from build123d import *

# Parameters (mm, degrees)
F0_W      = 101.61
F0_H      = 146
F1_DEPTH  = 1
F3_W      = 2
F3_H      = 146
F3_H_2    = 43.5
F4_DEPTH  = 9
F5_W      = 97.61
F5_H      = 5
F6_DEPTH  = 3
F9_W      = 5.5
F9_H      = 6
F10_DEPTH = 9
F11_D     = 2.7051
F12_D     = 3.7973


with BuildPart() as f1:
    # F0 (on Top) → F1 (new body)
    with BuildSketch(Plane.XY):
        with Locations((-50.805, -73)):
            Rectangle(F0_W, F0_H)
    extrude(amount=-F1_DEPTH)

    # F3 (on Top) → F4 (join)
    with BuildSketch(Plane.XY):
        with Locations((-100.61, -73)):
            Rectangle(F3_W, F3_H)
        with Locations((-1, -124.25)):
            Rectangle(F3_W, F3_H_2)
    extrude(amount=F4_DEPTH)

    # F5 (on face) → F6 (join)
    with BuildSketch(Plane.XY):
        with Locations((-50.805, -105)):
            Rectangle(F5_W, F5_H)
    extrude(amount=F6_DEPTH)

    # F9 (on face) → F10 (join, through all)
    with BuildSketch(Plane.XY):
        with Locations((-98.86, -130.3)):
            Rectangle(F9_W, F9_H)
        with Locations((-98.86, -70.11)):
            Rectangle(F9_W, F9_H)
        with Locations((-98.86, -28.5)):
            Rectangle(F9_W, F9_H)
        with Locations((-2.75, -130.3)):
            Rectangle(F9_W, F9_H)
    extrude(amount=F10_DEPTH)

    # F11 (through all)
    with Locations(Plane(origin=(-101.61, 0, 0), x_dir=(0, -1, 0), z_dir=(-1, 0, 0))):
        with Locations((28.5, 5.35), (70.11, 5.35), (130.3, 5.35)):
            Hole(F11_D / 2)

    # F12 (through all)
    with Locations(Plane.XY):
        with Locations((-65.785, -90.6), (-4.065, -90.6), (-4.065, -14), (-65.785, -14)):
            Hole(F12_D / 2)


solid = f1.part
The model under review builds one solid part; all positions refer to its coordinate system, in mm. A direction names the side the tool comes from. Round coordinates to 2 decimals unless told otherwise and drop trailing zeros. Order: outer loops, then holes, each group sorted by start corner. A loop starts at its lowest first (then second) coordinate and runs counter-clockwise, first axis right, second up. Notation, with made-up numbers: (-20.75, 56.5) -> (31.25, 56.5) arc R26 cw to (31.25, 70.5) -> close; hole circle Ø1 at (77, 45.5). An arc over 180 degrees is marked (long way). Use CSV: the item, a comma, the result in double quotes. Start each with the question number.
(1) Consider section B-B on x = -65.5. Write out the cut boundary in (y, z).
(2) Consider section C-C on y = -112. Write out the cut boundary in (x, z), and give its area (3 significant figures).
(3) Tool access review of faces 5 (the face through (-98, -73.11, 4)), 6 (the face through (-98, -25.5, 4)), 7 (the face through (-2, -115, 4)): name each direction out of +Z, -Z, +X, -X, +Y, -Y from which nothing blocks a thin tool from reaching the whole face with its end or side.
(4) Insertion check: pin 1 (1.5 mm diameter, centred on y = -76, z = 8, fed in from +X); pin 2 (3.5 mm diameter, centred on y = -130.3, z = 5.35, fed in from +X); pin 3 (1 mm diameter, centred on x = -97.5, z = 3.5, fed in from +Y); pin 4 (2.5 mm diameter, centred on y = -70.11, z = 5.35, fed in from +X). Each pin has a flat end and moves straight along its axis. Give the tip position at first contact, or say it passes through.
(5) Consider section D-D on x = -50.5. Write out the cut boundary in (y, z).
(6) Wall thickness on probe 1 along X at (y, z) = (-90.6, -0.7); probe 2 along Z at (x, y) = (-4, -130); probe 3 along X at (y, z) = (-52.5, 7): over which ranges is each line inside the solid? List them lowest first. Write a range as from..to.
(7) Consider section A-A on y = -90.6. Write out the cut boundary in (x, z), and give its area (3 significant figures).
(8) Mouldability with a two-part tool opening along X and no side actions: class faces 1 (the face through (-98.82, -129.01, 5.76)), 2 (the face through (-2, -140, 4)), 3 (the face through (-51, -126, 0)), 4 (the face through (-101.61, -74, 4)) as pulls with the +X half, pulls with the -X half, needs draft (parallel to the pull), parting line crosses it, or undercut.
Responses:
1,outline,"(-146, -1) -> (-92.48, -1) -> (-92.48, 0) -> (-102.5, 0) -> (-102.5, 3) -> (-107.5, 3) -> (-107.5, 0) -> (-146, 0) -> close; (-88.72, -1) -> (-15.88, -1) -> (-15.88, 0) -> (-88.72, 0) -> close; (-12.12, -1) -> (0, -1) -> (0, 0) -> (-12.12, 0) -> close"
2,outline,"(-101.61, -1) -> (0, -1) -> (0, 9) -> (-2, 9) -> (-2, 0) -> (-99.61, 0) -> (-99.61, 9) -> (-101.61, 9) -> close"
2,area,"138 mm²"
3,face 5,"+Z, +X"
3,face 6,"+Z, +X, +Y"
3,face 7,"+Z"
4,pin 1,"x = -99.61"
4,pin 2,"x = 0"
4,pin 3,"y = -25.5"
4,pin 4,"through"
5,outline,"(-146, -1) -> (0, -1) -> (0, 0) -> (-102.5, 0) -> (-102.5, 3) -> (-107.5, 3) -> (-107.5, 0) -> (-146, 0) -> close"
6,probe 1,"-101.61..-67.68, -63.89..-5.96, -2.17..0"
6,probe 2,"-1..4.03, 6.67..9"
6,probe 3,"-101.61..-99.61"
7,outline,"(-101.61, -1) -> (-67.68, -1) -> (-67.68, 0) -> (-99.61, 0) -> (-99.61, 9) -> (-101.61, 9) -> close; (-63.89, -1) -> (-5.96, -1) -> (-5.96, 0) -> (-63.89, 0) -> close; (-2.17, -1) -> (0, -1) -> (0, 0) -> (-2.17, 0) -> close"
7,area,"112 mm²"
8,face 1,"needs draft"
8,face 2,"undercut"
8,face 3,"undercut"
8,face 4,"pulls with the -X half"
